Model file for the job. Use its own axes, mm. A direction names the side the tool comes from. Round coordinates to 2 decimals unless told otherwise and drop trailing zeros. Order: outer loops, then holes, each group sorted by start corner. A loop starts at its lowest first (then second) coordinate and runs counter-clockwise, first axis right, second up. Notation, with made-up numbers: (57.25, 16) - (88.25, 16) arc R23 cw to (88.25, 40) - close; hole circle Ø11 at (79, 88). An arc over 180 degrees is marked (long way). Write item = value, one per line.
```python
from build123d import *

# Parameters (mm, degrees)
SKETCH1_W           = 137.961167182
SKETCH1_H           = 137.961167182
SKETCH1_R           = 3.175
BOSS_EXTRUDE1_DEPTH = 19.05
FILLET1_R           = 6.35
FILLET2_R           = 6.35


with BuildPart() as part:
    # Sketch1 → Boss-Extrude1 (new body)
    with BuildSketch(Plane(origin=(0, 0, 0), x_dir=(1, 0, 0), z_dir=(0, 1, 0))):
        Rectangle(SKETCH1_W, SKETCH1_H)
        Polygon((-61.63707698, -60.545979349), (-61.63707698, -15.874596852), (-56.280583591, -15.874596852), (-56.280583591, 56.280583591), (56.280583591, 56.280583591), (56.280583591, -56.280583591), (-47.38767698, -56.280583591), (-47.38767698, -60.545979349), align=None, mode=Mode.SUBTRACT)
        with Locations(Location((62.630583591, -62.630583591, 0), (0, 0, 90))):
            Circle(SKETCH1_R, mode=Mode.SUBTRACT)
        with Locations(Location((-62.630583591, 62.630583591, 0), (0, 0, 90))):
            Circle(SKETCH1_R, mode=Mode.SUBTRACT)
        with Locations(Location((62.630583591, 62.630583591, 0), (0, 0, 90))):
            Circle(SKETCH1_R, mode=Mode.SUBTRACT)
    extrude(amount=BOSS_EXTRUDE1_DEPTH)

    # Fillet1
    fillet1_edges = [part.edges().sort_by_distance(p)[0] for p in [
        (68.980583591, 9.525, -68.980583591),
        (68.980583591, 9.525, 68.980583591),
        (-68.980583591, 9.525, 68.980583591),
        (-68.980583591, 9.525, -68.980583591),
    ]]
    fillet(fillet1_edges, radius=FILLET1_R)

    # Fillet2
    # the kernel refuses this fillet: 6.35 mm, written as the material it takes off along each edge
    with BuildSketch(Plane(origin=(-56.280583591, -15.679493896, 15.874596852), x_dir=(-1, 0, 0), z_dir=(0, 1, 0))) as fillet2_piece_1:
        with BuildLine():
            CenterArc((6.35, -6.271797558), FILLET2_R, 99.001349837, 80.998650163)
            Line((0, -6.271797558), (-0.127, -6.271797558))
            Line((-0.127, -6.271797558), (-0.127, 0))
            Line((-0.127, 0), (0, 0.127))
            ThreePointArc((0, 0.127), (2.678246694, 0.127), (5.336623257, 0.125435951))
            Line((5.336623257, 0.125435951), (5.356493389, 0))
        make_face()
    extrude(amount=50.408987792, mode=Mode.SUBTRACT)
    with BuildSketch(Plane(origin=(-47.38767698, -14.99519197, 56.280583591), x_dir=(1, 0, 0), z_dir=(0, 1, 0))) as fillet2_piece_2:
        with BuildLine():
            CenterArc((5.998076788, -6.35), FILLET2_R, 90, 70.835337627)
            Line((0, -4.265395758), (-0.119961536, -4.223703673))
            ThreePointArc((-0.119961536, -4.223703673), (-0.127, -2.132697879), (-0.127, 0))
            Line((-0.127, 0), (0, 0.127))
            Line((0, 0.127), (5.998076788, 0.127))
            Line((5.998076788, 0.127), (5.998076788, 0))
        make_face()
    extrude(amount=49.04038394, mode=Mode.SUBTRACT)


solid = part.part
```
1) 3-axis set-ups, long thin cutter, end or side, ignore diameter. For faces 1 (the face through (-1, 9, 68.981)), 2 (the face through (-54, 9, 60.546)): which of +Z, -Z, +X, -X, +Y, -Y reach the whole face in a straight line?
Conclusion:
face_1 = +Z, +X, -X, +Y, -Y
face_2 = +Y, -Y
2) Wall check: line 1 along X through (y, z) = (4.75, 7); line 2 along X through (y, z) = (15, 41). Give the ranges that are in metal, low to high.
Conclusion:
line_1 = -68.98 to -56.28, 56.28 to 68.98
line_2 = -68.98 to -61.64, 56.28 to 68.98
3) Mould opens along X. For faces 3 (the face through (67.07, 9.66, -67.17)), 4 (the face through (-1, 0, 60)), 5 (the face through (59.483, 9.392, -62.217)) say: +X half, -X half, draft (parallel to the pull), parting line (faces both ways), or undercut.
Conclusion:
face_3 = +X half
face_4 = draft
face_5 = undercut
4) Cut at B-B (y = 9.5). Write the cut outline in (x, z) (3 decimals), and give its area (3 significant figures).
Conclusion:
outline = (-68.981, -62.631) arc R6.35 ccw to (-62.631, -68.981) - (62.631, -68.981) arc R6.35 ccw to (68.981, -62.631) - (68.981, 62.631) arc R6.35 ccw to (62.631, 68.981) - (-62.631, 68.981) arc R6.35 ccw to (-68.981, 62.631) - close; hole circle Ø6.35 at (-62.631, -62.631); hole (-61.637, 15.875) arc R6.35 cw to (-56.281, 9.603) - (-56.281, -56.281) - (56.281, -56.281) - (56.281, 56.281) - (-41.39, 56.281) arc R6.35 cw to (-47.388, 60.546) - (-61.637, 60.546) - close; hole circle Ø6.35 at (62.631, -62.631); hole circle Ø6.35 at (62.631, 62.631)
area = 5,940 mm^2
5) Cut at A-A (x = 46). Write the cut outline in (y, z), and give its area (3 significant figures).
Conclusion:
outline = (0, -68.98) - (19.05, -68.98) - (19.05, -56.28) - (0, -56.28) - close; (0, 56.28) - (19.05, 56.28) - (19.05, 68.98) - (0, 68.98) - close
area = 484 mm^2
6) Flat gauge pin, fed straight in: pin 1 Ø5 at (x, z) = (62.63, -62.63) entering from -Y. Where does the tip first touch, or does it go through?
Conclusion:
pin_1 = through
7) Cut at C-C (z = 3). Write the cut outline in (x, y), and give its area (3 significant figures).
Conclusion:
outline = (-68.98, 0) - (-56.28, 0) - (-56.28, 19.05) - (-68.98, 19.05) - close; (56.28, 0) - (68.98, 0) - (68.98, 19.05) - (56.28, 19.05) - close
area = 484 mm^2
